Here's the drawing with two shaded views (mm, measured from the low corner). I have some questions. A direction names the side the tool comes from. Round coordinates to 2 decimals unless told otherwise and drop trailing zeros. Loops run counter-clockwise (first coordinate to the right, second up) from the corner with the lowest first, then second, coordinate; pieces in that order, holes last.
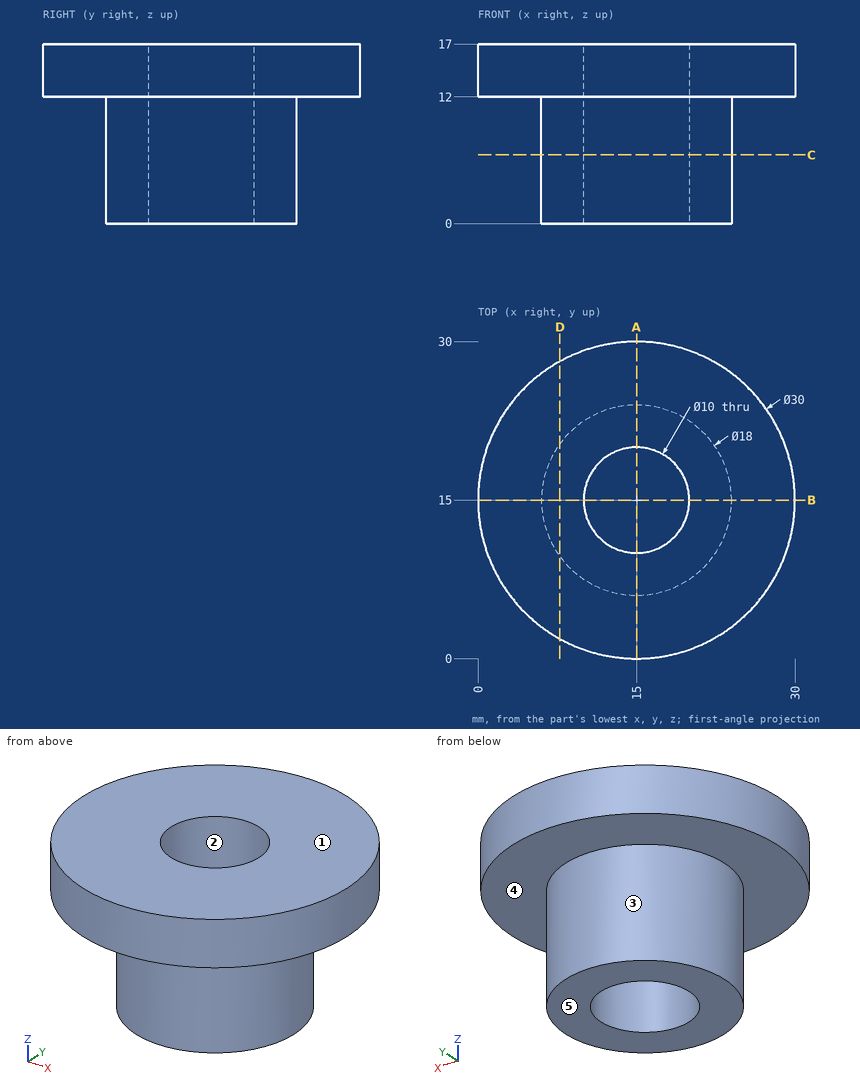
(1) Will these pins go through, and if not, where does the flat tip stop? P1, Ø1, axis at x = 25, y = 14.5, coming from the -Z side; P2, Ø1.5, axis at y = 18, z = 7.5, coming from the +X side; P3, Ø2, axis at x = 20.5, z = 2, coming from the +Y side; P4, Ø9, axis at x = 15, y = 15, coming from the +Z side.
Worked answers:
P1: stops at z = 12
P2: stops at x = 23.71
P3: stops at y = 22.79
P4: passes through
(2) If we section it at D-D, the plane x = 7.75: List the corners of the cut face in (y, z) for me, then the cut area to 3 significant figures.
Worked answers:
outline: (1.87, 12) - (9.67, 12) - (9.67, 0) - (20.33, 0) - (20.33, 12) - (28.13, 12) - (28.13, 17) - (1.87, 17) - close
area: 259 mm2
(3) If we section it at C-C, the plane z = 6.5: List the corners of the cut face in (x, y) for me.
Worked answers:
outline: circle Ø18 at (15, 15); hole circle Ø10 at (15, 15)
(4) If we mould it in two halves opening along X, with no side actions, what happens to the marked faces 1, 2 and 3? For each: released by +X, released by -X, zero draft, split by the parting line, or undercut.
Worked answers:
face 1: zero draft
face 2: undercut
face 3: split by the parting line
(5) If we section it at A-A, the plane x = 15: List the corners of the cut face in (y, z) for me, then the cut area to 3 significant figures.
Worked answers:
outline: (0, 12) - (6, 12) - (6, 0) - (10, 0) - (10, 17) - (0, 17) - close; (20, 0) - (24, 0) - (24, 12) - (30, 12) - (30, 17) - (20, 17) - close
area: 196 mm2
(6) For the marked faces 4 and 5, which set-ups out of +Z, -Z, +X, -X, +Y, -Y let a thin tool reach every point of the face, with its end or its side?
Worked answers:
face 4: -Z
face 5: -Z, +X, -X, +Y, -Y
(7) If I drill on line 1 (Y direction, x = 15, z = 6.25); line 2 (Z direction, x = 23.5, y = 21.5); line 3 (X direction, y = 13, z = 9), over which ranges is the centre line in solid material (lowest first)?
Worked answers:
line 1: y = 6 to 10, 20 to 24
line 2: z = 12 to 17
line 3: x = 6.23 to 10.42, 19.58 to 23.77
